Can you work these out from the model? Positions are in its coordinate system, mm. A direction names the side the tool comes from. Coordinates: 2 decimals unless noted, no trailing zeros. Loops run counter-clockwise (first coordinate to the right, second up) from the corner with the lowest first, then second, coordinate; pieces in that order, holes last. Notation, with made-up numbers: (-26.75, 62.5) -> (6.25, 62.5) arc R20 ccw to (6.25, 100.5) -> close; hole circle Ø3 at (26, 17). An arc over 180 degrees is marked (long way). Put each result on its own line as item: value. Start each with the question number.
Item 1: For faces 4 (the flat face through (9, -5, 50)), 5 (the flat face through (2, 10, 39)), 6 (the cylindrical face through (2.308, 10.14, 2.676)), which set-ups out of +Z, -Z, +X, -X, +Y, -Y let a thin tool reach every point of the face, with its end or its side?
Item 2: If we section it at C-C on y = 1: Please give me the cut outline in (x, z).
Item 3: If we section it at B-B on x = 9.5: Please give me the cut outline in (y, z).
Item 4: Please list where these lines run through material, in increasing order: L1, parallel to Y at x = 9.5, z = 53.5; L2, parallel to X at y = 16.5, z = 11; L3, parallel to Y at x = 13, z = 5. Write a range as from..to.
Item 5: We'd pull the mould along Y, two halves only. Please class faces 1 (the cylindrical face through (9.066, 25.548, 55.07)), 2 (the flat face through (8, 10, -10)), 3 (the cylindrical face through (9.6, 34.1, 50.86)): pulls with the +Y half, pulls with the -Y half, needs draft (parallel to the pull), parting line crosses it, or undercut.
Item 6: Will these pins go through, and if not, where does the flat tip stop? P1, Ø4.5, axis at x = 6, y = -9, coming from the -Z side; P2, Ø12, axis at y = 1.5, z = 13.5, coming from the -X side; P3, Ø4.5, axis at x = 2, z = 0, coming from the +Y side; P4, Ø5, axis at y = 24.5, z = -0.5, coming from the +X side.
Item 7: If we section it at D-D on z = 28: Please give me the cut outline in (x, y).
Item 8: If we section it at A-A on y = -7.5: Please give me the cut outline in (x, z).
```python
from build123d import *

# Parameters (mm, degrees)
BOSS_EXTRUDE1_DEPTH = 20
SKETCH2_W           = 15
SKETCH2_H           = 15
SKETCH2_R           = 2
BOSS_EXTRUDE2_DEPTH = 10
FILLET1_R           = 3


with BuildPart() as part:
    # Sketch1 → Boss-Extrude1 (new body)
    with BuildSketch(Plane(origin=(0, 0, 0), x_dir=(1, 0, 0), z_dir=(0, 1, 0))):
        with BuildLine():
            Line((0, 0), (-13, 0))
            Line((-13, 0), (-13, 7))
            Line((-13, 7), (2, 10))
            Line((2, 10), (17, 10))
            Line((17, 10), (17, -60))
            Line((17, -60), (2, -60))
            Line((2, -60), (2, -2))
            ThreePointArc((2, -2), (3.414213562, 1.414213562), (0, 0))
        make_face()
    extrude(amount=BOSS_EXTRUDE1_DEPTH)

    # Sketch2 → Boss-Extrude2 (add)
    with BuildSketch(Plane.XY.offset(60)):
        with Locations((9.5, 27.5)):
            Rectangle(SKETCH2_W, SKETCH2_H)
        with Locations((9.5, 27.5)):
            Circle(SKETCH2_R, mode=Mode.SUBTRACT)
        with Locations((9.5, -7.5)):
            Rectangle(SKETCH2_W, SKETCH2_H)
        with Locations((9.5, -7.5)):
            Circle(SKETCH2_R, mode=Mode.SUBTRACT)
    extrude(amount=-BOSS_EXTRUDE2_DEPTH)

    # Fillet1
    fillet1_edges = [part.edges().sort_by_distance(p)[0] for p in [
        (0, 10, 0),
        (-13, 10, -7),
        (2, 10, -10),
        (17, 10, -10),
        (2, 10, 2),
        (9.5, 35, 50),
        (9.5, 20, 50),
        (9.5, 0, 50),
        (9.5, -15, 50),
    ]]
    fillet(fillet1_edges, radius=FILLET1_R)


solid = part.part
```
Solutions:
1. face 4: -Z, +X, -X, -Y
1. face 5: +Z, -X, +Y, -Y
1. face 6: -X, +Y, -Y
2. outline: (-13, -4.54) arc R3 ccw to (-10.59, -7.48) -> (1.71, -9.94) arc R3 ccw to (2.3, -10) -> (14, -10) arc R3 ccw to (17, -7) -> (17, 60) -> (2, 60) -> (2, 4) arc R3 ccw to (3.2, 1.6) arc R2 cw (long way) to (0.4, -1.2) arc R3 ccw to (-2, 0) -> (-13, 0) -> close
3. outline: (-15, 53) arc R3 ccw to (-12, 50) -> (-9.5, 50) -> (-9.5, 60) -> (-15, 60) -> close; (-5.5, 50) -> (-3, 50) arc R3 cw to (0, 47) -> (0, -10) -> (20, -10) -> (20, 47) arc R3 cw to (23, 50) -> (25.5, 50) -> (25.5, 60) -> (-5.5, 60) -> close; (29.5, 50) -> (32, 50) arc R3 ccw to (35, 53) -> (35, 60) -> (29.5, 60) -> close
4. L1: -15..-9.5, -5.5..25.5, 29.5..35
4. L2: 2..17
4. L3: 0..20
5. face 1: undercut
5. face 2: needs draft
5. face 3: pulls with the +Y half
6. P1: z = 50
6. P2: x = 2
6. P3: y = 20
6. P4: through
7. outline: (2, 0) -> (17, 0) -> (17, 20) -> (2, 20) -> close
8. outline: (2, 50) -> (7.5, 50) -> (7.5, 60) -> (2, 60) -> close; (11.5, 50) -> (17, 50) -> (17, 60) -> (11.5, 60) -> close
